```python
from build123d import *

# Parameters (mm, degrees)
SKETCH1_R           = 17.25
BOSS_EXTRUDE1_DEPTH = 15
SKETCH2_R           = 6
BOSS_EXTRUDE2_DEPTH = 4.5
BOSS_EXTRUDE3_DEPTH = 6.9
SKETCH4_W           = 33
SKETCH4_H           = 33
BOSS_EXTRUDE4_DEPTH = 1.6
FILLET1_R           = 3
SKETCH9_W           = 12
SKETCH9_H           = 10
BOSS_EXTRUDE6_DEPTH = 5.5
SKETCH10_R          = 1.25
CUT_EXTRUDE1_DEPTH  = 4
SKETCH11_R          = 3.1
BOSS_EXTRUDE7_DEPTH = 1.4
FILLET2_R           = 2
SKETCH12_R          = 3.25
CUT_EXTRUDE2_DEPTH  = 12


with BuildPart() as part:
    # Sketch1 → Boss-Extrude1 (new body)
    with BuildSketch(Plane(origin=(0, 0, 0), x_dir=(1, 0, 0), z_dir=(0, 1, 0))):
        with Locations(Location((0, 0, 0), (0, 0, 270))):
            Circle(SKETCH1_R)
    extrude(amount=BOSS_EXTRUDE1_DEPTH)

    # Sketch2 → Boss-Extrude2 (add)
    with BuildSketch(Plane.XZ):
        with Locations(Location((0, 0, 0), (0, 0, 270))):
            Circle(SKETCH2_R)
    extrude(amount=BOSS_EXTRUDE2_DEPTH)

    # Sketch3 → Boss-Extrude3 (add)
    with BuildSketch(Plane.XZ):
        Polygon((-6.844188762, 0), (-8.172094381, 2.3), (-10.827905619, 2.3), (-12.155811238, 0), (-10.827905619, -2.3), (-8.172094381, -2.3), align=None)
        Polygon((12.155811238, 0), (10.827905619, 2.3), (8.172094381, 2.3), (6.844188762, 0), (8.172094381, -2.3), (10.827905619, -2.3), align=None)
    extrude(amount=BOSS_EXTRUDE3_DEPTH)

    # Sketch4 → Boss-Extrude4 (add)
    with BuildSketch(Plane.XZ.offset(6.9)):
        Rectangle(SKETCH4_W, SKETCH4_H)
        with BuildLine():
            Line((-13.116830791, -10.924799769), (-10.995510447, -8.803479426))
            ThreePointArc((-10.995510447, -8.803479426), (-8.803479426, -8.803479426), (-8.803479426, -10.995510447))
            Line((-8.803479426, -10.995510447), (-10.924799769, -13.116830791))
            ThreePointArc((-10.924799769, -13.116830791), (-13.116830791, -13.116830791), (-13.116830791, -10.924799769))
        make_face(mode=Mode.SUBTRACT)
        with BuildLine():
            Line((-13.116830791, 10.924799769), (-10.995510447, 8.803479426))
            ThreePointArc((-10.995510447, 8.803479426), (-8.803479426, 8.803479426), (-8.803479426, 10.995510447))
            Line((-8.803479426, 10.995510447), (-10.924799769, 13.116830791))
            ThreePointArc((-10.924799769, 13.116830791), (-13.116830791, 13.116830791), (-13.116830791, 10.924799769))
        make_face(mode=Mode.SUBTRACT)
        with BuildLine():
            Line((13.116830791, -10.924799769), (10.995510447, -8.803479426))
            ThreePointArc((10.995510447, -8.803479426), (8.803479426, -8.803479426), (8.803479426, -10.995510447))
            Line((8.803479426, -10.995510447), (10.924799769, -13.116830791))
            ThreePointArc((10.924799769, -13.116830791), (13.116830791, -13.116830791), (13.116830791, -10.924799769))
        make_face(mode=Mode.SUBTRACT)
        with BuildLine():
            Line((13.116830791, 10.924799769), (10.995510447, 8.803479426))
            ThreePointArc((10.995510447, 8.803479426), (8.803479426, 8.803479426), (8.803479426, 10.995510447))
            Line((8.803479426, 10.995510447), (10.924799769, 13.116830791))
            ThreePointArc((10.924799769, 13.116830791), (13.116830791, 13.116830791), (13.116830791, 10.924799769))
        make_face(mode=Mode.SUBTRACT)
    extrude(amount=BOSS_EXTRUDE4_DEPTH)

    # Fillet1
    fillet1_edges = [part.edges().sort_by_distance(p)[0] for p in [
        (-16.5, -7.7, -16.5),
        (16.5, -7.7, -16.5),
        (16.5, -7.7, 16.5),
        (-16.5, -7.7, 16.5),
    ]]
    fillet(fillet1_edges, radius=FILLET1_R)

    # Sketch9 → Boss-Extrude6 (add)
    with BuildSketch(Plane.XZ.offset(8.5)):
        with Locations((0, 9)):
            Rectangle(SKETCH9_W, SKETCH9_H)
        with Locations((0, -9)):
            Rectangle(SKETCH9_W, SKETCH9_H)
    extrude(amount=BOSS_EXTRUDE6_DEPTH)

    # Sketch10 → Cut-Extrude1 (cut)
    with BuildSketch(Plane(origin=(0, 15, 0), x_dir=(1, 0, 0), z_dir=(0, 1, 0))):
        with Locations(Location((0, 8, 0), (0, 0, 270))):
            Circle(SKETCH10_R)
        with Locations(Location((8, 0, 0), (0, 0, 270))):
            Circle(SKETCH10_R)
        with Locations(Location((0, -8, 0), (0, 0, 270))):
            Circle(SKETCH10_R)
        with Locations(Location((-8, 0, 0), (0, 0, 270))):
            Circle(SKETCH10_R)
    extrude(amount=-CUT_EXTRUDE1_DEPTH, mode=Mode.SUBTRACT)

    # Sketch11 → Boss-Extrude7 (add)
    with BuildSketch(Plane.XZ.offset(8.5)):
        with Locations(Location((-9.5, 0, 0), (0, 0, 270))):
            Circle(SKETCH11_R)
        with Locations(Location((9.5, 0, 0), (0, 0, 270))):
            Circle(SKETCH11_R)
    extrude(amount=BOSS_EXTRUDE7_DEPTH)

    # Fillet2
    # the kernel refuses this fillet: 2 mm, written as the material it takes off along each edge
    with BuildSketch(Plane(origin=(-9.5, -9.9, 0), x_dir=(0, 0, -1), z_dir=(-1, 0, 0))) as fillet2_piece_1:
        with BuildLine():
            CenterArc((1.192121597, -2), FILLET2_R, 17.457603124, 72.542396876)
            Line((1.192121597, 0), (1.192121597, 0.04))
            Line((1.192121597, 0.04), (3.1, 0.04))
            Line((3.1, 0.04), (3.14, 0))
            ThreePointArc((3.14, 0), (3.14, -0.7), (3.138157568, -1.388))
            Line((3.138157568, -1.388), (3.1, -1.4))
        make_face()
    revolve(axis=Axis((-9.5, -9.9, 0), (0, -1, 0)), mode=Mode.SUBTRACT)
    with BuildSketch(Plane(origin=(9.5, -9.9, 0), x_dir=(0, 0, -1), z_dir=(-1, 0, 0))) as fillet2_piece_2:
        with BuildLine():
            CenterArc((1.192121597, -2), FILLET2_R, 17.457603124, 72.542396876)
            Line((1.192121597, 0), (1.192121597, 0.04))
            Line((1.192121597, 0.04), (3.1, 0.04))
            Line((3.1, 0.04), (3.14, 0))
            ThreePointArc((3.14, 0), (3.14, -0.7), (3.138157568, -1.388))
            Line((3.138157568, -1.388), (3.1, -1.4))
        make_face()
    revolve(axis=Axis((9.5, -9.9, 0), (0, -1, 0)), mode=Mode.SUBTRACT)

    # Sketch12 → Cut-Extrude2 (cut)
    with BuildSketch(Plane(origin=(0, 15, 0), x_dir=(1, 0, 0), z_dir=(0, 1, 0))):
        with Locations(Location((0, 0, 0), (0, 0, 270))):
            Circle(SKETCH12_R)
    extrude(amount=-CUT_EXTRUDE2_DEPTH, mode=Mode.SUBTRACT)


solid = part.part
```
Can you work these out from the model? Positions are in its coordinate system, mm. A direction names the side the tool comes from. Give positions to 0.01 mm unless a question says otherwise; leave off trailing zeros. Write each loop counter-clockwise with the first axis right and the second up, starting at its lowest first coordinate (ties: lowest second). Pieces come first, ordered by that corner, then holes. Notation, with made-up numbers: (43, 86) -> (57, 86) arc R23 ccw to (57, 123) -> close; hole circle Ø8 at (26, 34). An arc over 180 degrees is marked (long way). One line per item, written item: value.
Q1. Imagine slicing it at D-D on y = 1. Please give me the cut outline in (x, z).
Results found:
outline: circle Ø34.5 at (0, 0)
Q2. We'd pull the mould along Z, two halves only. Please class faces 1 (the face through (10, -3, 2.3)), 2 (the face through (-10, -3, -2.3)), 3 (the face through (0.758, 7.395, -17.233)), 4 (the face through (9.85, -7.69, -12.04)): +Z half, -Z half, draft (parallel to the pull), parting line (faces both ways), or undercut.
Results found:
face 1: +Z half
face 2: -Z half
face 3: parting line
face 4: undercut
Q3. Please list where these lines run through material, in increasing order: line 1 (X direction, y = 14.2, z = 0); line 2 (Y direction, x = 7.5, z = 4.5); line 3 (Y direction, x = 1.5, z = 11.5). Write a range as [from, to].
Results found:
line 1: x = [-17.25, -9.25], [-6.75, -3.25], [3.25, 6.75], [9.25, 17.25]
line 2: y = [-8.5, -6.9], [0, 15]
line 3: y = [-14, -6.9], [0, 15]
Q4. Imagine slicing it at C-C on z = -7.5. Please give me the cut outline in (x, y), and give its area (3 significant figures).
Results found:
outline: (-16.5, -8.5) -> (-6, -8.5) -> (-6, -14) -> (6, -14) -> (6, -8.5) -> (16.5, -8.5) -> (16.5, -6.9) -> (-16.5, -6.9) -> close; (-15.53, 0) -> (15.53, 0) -> (15.53, 15) -> (1.15, 15) -> (1.15, 11) -> (-1.15, 11) -> (-1.15, 15) -> (-15.53, 15) -> close
area: 576 mm^2
Q5. Imagine slicing it at B-B on y = 12. Please give me the cut outline in (x, z).
Results found:
outline: circle Ø34.5 at (0, 0); hole circle Ø2.5 at (-8, 0); hole circle Ø6.5 at (0, 0); hole circle Ø2.5 at (0, -8); hole circle Ø2.5 at (0, 8); hole circle Ø2.5 at (8, 0)
Q6. For P1, Ø1.6, axis at x = -1, y = -12.5, coming from the +Z side; P2, Ø0.8, axis at x = -5, y = -7.5, coming from the +Z side; P3, Ø0.5, axis at y = -7.5, z = -0.5, coming from the -X side, each with a flat end and sliding along its axis, tell me the tip position at first contact or that it passes through.
Results found:
P1: stops at z = 14
P2: stops at z = 16.5
P3: stops at x = -16.5
Q7. Which directions (+Z, -Z, +X, -X, +Y, -Y) give clear straight access to the entire face, cutting with the end or side of a thin tool? Please do faces 5 (the face through (-8.83, -7.69, -8.78)), 6 (the face through (0.05, 13.03, 6.75)), 7 (the face through (6, -11, -9)), 8 (the face through (0, -11, -4)).
Results found:
face 5: -Y
face 6: +Y
face 7: +Z, -Z, +X, -Y
face 8: +X, -X, -Y
